The figure shows three views and two pictorial views of one solid part (mm, origin at its lowest corner). Answer the questions. Coordinates: 2 decimals unless noted, no trailing zeros. Order: outer loops, then holes, each group sorted by start corner. A loop starts at its lowest first (then second) coordinate and runs counter-clockwise, first axis right, second up. Notation, with made-up numbers: (-7, -17.5) - (22, -17.5) arc R34 cw to (22, 16.5) - close; hole circle Ø7 at (66, 44.5). An arc over 180 degrees is marked (long way). Use one line per item in the form item = value.
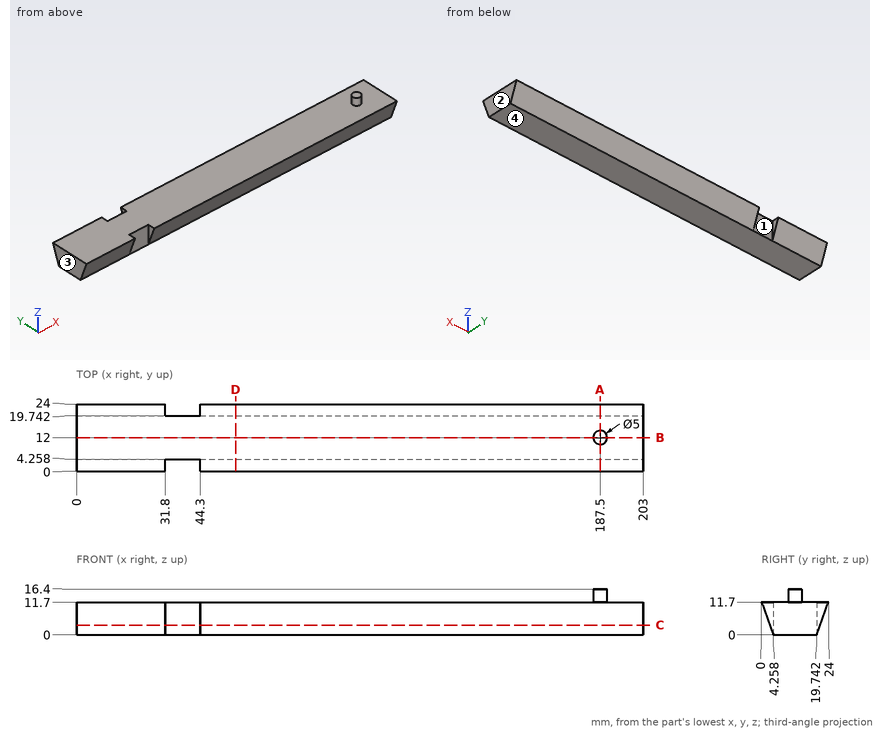
(1) Section A-A, the plane x = 187.5 is taken. Write down the section's boundary in (y, z).
Answer list:
outline = (0, 11.7) - (4.26, 0) - (19.74, 0) - (24, 11.7) - (14.5, 11.7) - (14.5, 16.4) - (9.5, 16.4) - (9.5, 11.7) - close
(2) Section B-B, the plane y = 12 is taken. Write down the section's boundary in (x, z), then the cut area to 3 significant figures.
Answer list:
outline = (0, 0) - (203, 0) - (203, 11.7) - (190, 11.7) - (190, 16.4) - (185, 16.4) - (185, 11.7) - (0, 11.7) - close
area = 2,400 mm2
(3) The mould has two halves that part along X. Classify the marked faces 1, 2, 3 and 4: +X half, -X half, draft (parallel to the pull), parting line (faces both ways), or undercut.
Answer list:
face_1 = undercut
face_2 = +X half
face_3 = -X half
face_4 = draft
(4) Given pin 1 Ø3.5 at (x, z) = (39, 4.5) entering from -Y; pin 2 Ø8 at (x, y) = (167.5, 5) entering from +Z; pin 3 Ø6 at (x, z) = (70.5, 12.5) entering from +Y, each flat-ended and moving along its own axis, determine where each tip first touches the part or whether it passes through.
Answer list:
pin_1 = 4.26
pin_2 = 11.7
pin_3 = 24
(5) Straight lines are drawn through the part: L1, parallel to X at y = 1.75, z = 7; L2, parallel to Z at x = 148.5, y = 5.75; L3, parallel to Y at x = 39, z = 6.5. For each, find the intervals that lie inside material, in ascending order.
Answer list:
L1 = 0 to 31.8, 44.3 to 203
L2 = 0 to 11.7
L3 = 4.26 to 19.74
(6) Section C-C, the plane z = 3.5 is taken. Write down the section's boundary in (x, y) (1 decimal), then the cut area to 3 significant figures.
Answer list:
outline = (0, 3) - (31.8, 3) - (31.8, 4.3) - (44.3, 4.3) - (44.3, 3) - (203, 3) - (203, 21) - (44.3, 21) - (44.3, 19.7) - (31.8, 19.7) - (31.8, 21) - (0, 21) - close
area = 3,630 mm2
(7) Section D-D, the plane x = 57 is taken. Write down the section's boundary in (y, z).
Answer list:
outline = (0, 11.7) - (4.26, 0) - (19.74, 0) - (24, 11.7) - close
